```python
from build123d import *

# Parameters (mm, degrees)
SKETCH1_R           = 3
SKETCH1_R_2         = 2
BOSS_EXTRUDE1_DEPTH = 5.5
BOSS_EXTRUDE2_DEPTH = 1.5
SKETCH3_R           = 2
CUT_EXTRUDE1_DEPTH  = 11.5
SKETCH4_R           = 1
CUT_EXTRUDE2_DEPTH  = 11.5
CHAMFER1_SIZE       = 1


with BuildPart() as part:
    # Sketch1 → Boss-Extrude1 (new body)
    with BuildSketch(Plane(origin=(0, 0, 0), x_dir=(1, 0, 0), z_dir=(0, 1, 0))):
        with Locations(Location((0, 0, 0), (0, 0, 270))):
            Circle(SKETCH1_R)
        with Locations(Location((0, 0, 0), (0, 0, 270))):
            Circle(SKETCH1_R_2, mode=Mode.SUBTRACT)
    extrude(amount=BOSS_EXTRUDE1_DEPTH)

    # Sketch2 → Boss-Extrude2 (add)
    with BuildSketch(Plane(origin=(0, 5.5, 0), x_dir=(1, 0, 0), z_dir=(0, 1, 0))):
        with BuildLine():
            Line((5.766281297, 3), (-5.766281297, 3))
            ThreePointArc((-5.766281297, 3), (-6.5, 0), (-5.766281297, -3))
            Line((-5.766281297, -3), (5.766281297, -3))
            ThreePointArc((5.766281297, -3), (6.5, 0), (5.766281297, 3))
        make_face()
    extrude(amount=BOSS_EXTRUDE2_DEPTH)

    # Sketch3 → Cut-Extrude1 (cut)
    with BuildSketch(Plane.XZ.offset(-5.5)):
        with Locations(Location((0, 0, 0), (0, 0, 90))):
            Circle(SKETCH3_R)
    extrude(amount=-CUT_EXTRUDE1_DEPTH, mode=Mode.SUBTRACT)

    # Sketch4 → Cut-Extrude2 (cut)
    with BuildSketch(Plane(origin=(0, 7, 0), x_dir=(1, 0, 0), z_dir=(0, 1, 0))):
        with Locations(Location((-4.75, 0, 0), (0, 0, 270))):
            Circle(SKETCH4_R)
        with Locations(Location((4.75, 0, 0), (0, 0, 270))):
            Circle(SKETCH4_R)
    extrude(amount=-CUT_EXTRUDE2_DEPTH, mode=Mode.SUBTRACT)

    # Chamfer1
    chamfer1_edges = [part.edges().sort_by_distance(p)[0] for p in [
        (0, 0, -2),
    ]]
    chamfer(chamfer1_edges, length=CHAMFER1_SIZE - 0.0001)  # a hair under: the kernel refuses the full size


solid = part.part
```
Input: part model. Units: mm. Frame: model coordinates. A direction names the side the tool comes from. Round coordinates to 2 decimals unless told otherwise and drop trailing zeros. Loops run counter-clockwise (first coordinate to the right, second up) from the corner with the lowest first, then second, coordinate; pieces in that order, holes last. Notation, with made-up numbers: M 18,43 L 53,43 A20 cw 53,53 Z; hole C 4,88 d10. An arc over 180 degrees is marked long. Answer in a Markdown table with one row per item. Add a question column.
1. Set-up query: faces 1 (the face through (5.74, 6.26, -0.13)), 2 (the face through (0.9, 2.71, 2.86)). Return all of +Z, -Z, +X, -X, +Y, -Y with unobstructed straight access to the full face (end or side cutting, diameter ignored); none if empty.
2. Ray query, probe 1 along X at (y, z) = (4.5, 0); probe 2 along X at (y, z) = (0.75, -0.25). Return the intervals inside material, ascending.
3. Mould query, pull axis X, two halves, no side actions, for faces 3 (the face through (0, 6, -3)), 4 (the face through (6.5, 6.2, 0)), 5 (the face through (-3.76, 6.26, -0.13)). Classes: released by +X, released by -X, zero draft, split by the parting line, or undercut.
4. Section D-D (y = 2.75). Output: boundary loops of the cut face in (x, z), and give its area (3 significant figures).
5. Section B-B (x = 4.75). Output: boundary loops of the cut face in (y, z), and give its area (3 significant figures).
6. Section A-A (z = 0). Give the number of separate pieces and of enclosed holes in the cut face, and give its area (3 significant figures).
7. Contact query for a flat-ended pin moving along its axis: pin 1 (3 mm diameter, centred on y = 3, z = -1, fed in from -X). Output: stop coordinate, or through.
8. Section C-C (y = 5.75). Output: boundary loops of the cut face in (x, z), and give its area (3 significant figures).
Values follow:
| question | item | result |
|---|---|---|
| 1 | face 1 | +Y, -Y |
| 1 | face 2 | -Y |
| 2 | probe 1 | -3 to -2, 2 to 3 |
| 2 | probe 2 | -2.99 to -2.24, 2.24 to 2.99 |
| 3 | face 3 | zero draft |
| 3 | face 4 | released by +X |
| 3 | face 5 | undercut |
| 4 | outline | C 0,0 d6; hole C 0,0 d4 |
| 4 | area | 15.7 mm^2 |
| 5 | outline | M 5.5,-3 L 7,-3 L 7,-1 L 5.5,-1 Z; M 5.5,1 L 7,1 L 7,3 L 5.5,3 Z |
| 5 | area | 6.00 mm^2 |
| 6 | separate pieces | 4 |
| 6 | enclosed holes | 0 |
| 6 | area | 17.5 mm^2 |
| 7 | pin 1 | x = -3 |
| 8 | outline | M -5.77,-3 L 5.77,-3 A6.5 ccw 5.77,3 L -5.77,3 A6.5 ccw Z; hole C -4.75,0 d2; hole C 0,0 d4; hole C 4.75,0 d2 |
| 8 | area | 56.3 mm^2 |
